```python
from build123d import *

# Parameters (mm, degrees)
F1_DEPTH = 1.7
F2_DEPTH = 7
F3_DEPTH = 22


with BuildPart() as f1:
    # F0 (on Top) → F1 (new body)
    with BuildSketch(Plane.XY):
        with BuildLine():
            Line((-22, -24), (-16, -24))
            Line((-16, -24), (-16, -14))
            ThreePointArc((-16, -14), (-11.313708, -2.686292), (0, 2))
            Line((0, 2), (128, 2))
            ThreePointArc((128, 2), (139.313708, -2.686292), (144, -14))
            Line((144, -14), (144, -24))
            Line((144, -24), (150, -24))
            Line((150, -24), (150, -14))
            ThreePointArc((150, -14), (143.556349, 1.556349), (128, 8))
            Line((128, 8), (0, 8))
            ThreePointArc((0, 8), (-15.556349, 1.556349), (-22, -14))
            Line((-22, -14), (-22, -24))
        make_face()
    extrude(amount=F1_DEPTH)

    # F0 (on Top) → F2 (join)
    with BuildSketch(Plane.XY):
        with BuildLine():
            ThreePointArc((-14, -14), (-9.899495, -4.100505), (0, 0))
            Line((0, 0), (128, 0))
            ThreePointArc((128, 0), (137.899495, -4.100505), (142, -14))
            Line((142, -14), (142, -24))
            Line((142, -24), (144, -24))
            Line((144, -24), (144, -14))
            ThreePointArc((144, -14), (139.313708, -2.686292), (128, 2))
            Line((128, 2), (0, 2))
            ThreePointArc((0, 2), (-11.313708, -2.686292), (-16, -14))
            Line((-16, -14), (-16, -24))
            Line((-16, -24), (-14, -24))
            Line((-14, -24), (-14, -14))
        make_face()
    extrude(amount=F2_DEPTH)

    # F0 (on Top) → F3 (join)
    with BuildSketch(Plane.XY):
        with BuildLine():
            Line((-24, -24), (-22, -24))
            Line((-22, -24), (-22, -14))
            ThreePointArc((-22, -14), (-15.556349, 1.556349), (0, 8))
            Line((0, 8), (128, 8))
            ThreePointArc((128, 8), (143.556349, 1.556349), (150, -14))
            Line((150, -14), (150, -24))
            Line((150, -24), (152, -24))
            Line((152, -24), (152, -14))
            ThreePointArc((152, -14), (144.970563, 2.970563), (128, 10))
            Line((128, 10), (0, 10))
            ThreePointArc((0, 10), (-16.970563, 2.970563), (-24, -14))
            Line((-24, -14), (-24, -24))
        make_face()
    extrude(amount=F3_DEPTH)


solid = f1.part
```
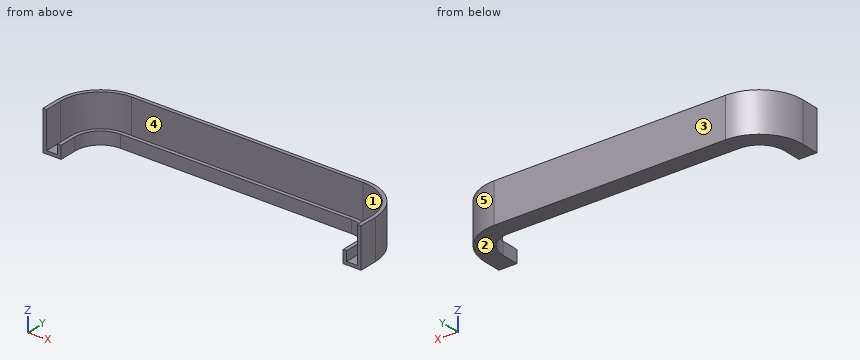
Geometry: final body of the model. Coordinates: model frame, mm. Face numbers are marked on the shaded views. A direction names the side the tool comes from. Coordinates: 2 decimals unless noted, no trailing zeros. Order: outer loops, then holes, each group sorted by start corner. A loop starts at its lowest first (then second) coordinate and runs counter-clockwise, first axis right, second up. Notation, with made-up numbers: M 88.5,-10 L 99.5,-10 A29 cw 99.5,18 Z; hole C 70,78 d6. An arc over 180 degrees is marked long. Answer in a Markdown table with one row per item. Add a question column.
Q1. Mould query, pull axis Y, two halves, no side actions, for the marked faces 1, 2 and 3. Classes: released by +Y, released by -Y, zero draft, split by the parting line, or undercut.
Q2. Section query D-D on y = -6. Return the cut outline in (x, z), and give its area (3 significant figures).
Q3. Reachability of the marked faces 4 and 5 from +Z, -Z, +X, -X, +Y, -Y: full face, straight path, thin tool, end or side. Return the list, or none.
Q4. Line query: L1, parallel to X at y = -14, z = 5; L2, parallel to X at y = -11, z = 6.5; L3, parallel to X at y = -21.5, z = 1. Output: solid intervals per line, ascending.
Q5. Section query A-A on y = -15.5. Return the cut outline in (x, z), and give its area (3 significant figures).
Q6. Section query C-C on x = 15. Return the cut outline in (y, z), and give its area (3 significant figures).
Q7. Section query B-B on z = 16.5. Return the cut outline in (x, y), and give its area (3 significant figures).
Q8. Contact query for flat-ended pins moving along their axis: P1, Ø1.5, axis at y = 3.5, z = 11.5, coming from the +X side; P2, Ø2, axis at y = 1, z = 19, coming from the +X side; P3, Ø6, axis at x = 72.5, z = 7, coming from the -Y side. Output: stop coordinate, or through.
Completed:
| question | item | result |
|---|---|---|
| 1 | face 1 | undercut |
| 1 | face 2 | zero draft |
| 1 | face 3 | released by +Y |
| 2 | outline | M -22.63,0 L -11.49,0 L -11.49,7 L -13.86,7 L -13.86,1.7 L -20.49,1.7 L -20.49,22 L -22.63,22 Z; M 139.49,0 L 150.63,0 L 150.63,22 L 148.49,22 L 148.49,1.7 L 141.86,1.7 L 141.86,7 L 139.49,7 Z |
| 2 | area | 150 mm2 |
| 3 | face 4 | +Z |
| 3 | face 5 | +Z, -Z, +X, +Y |
| 4 | L1 | x = -24 to -22, -16 to -14, 142 to 144, 150 to 152 |
| 4 | L2 | x = -23.81 to -21.79, -15.72 to -13.67, 141.67 to 143.72, 149.79 to 151.81 |
| 4 | L3 | x = -24 to -14, 142 to 152 |
| 5 | outline | M -24,0 L -14,0 L -14,7 L -16,7 L -16,1.7 L -22,1.7 L -22,22 L -24,22 Z; M 142,0 L 152,0 L 152,22 L 150,22 L 150,1.7 L 144,1.7 L 144,7 L 142,7 Z |
| 5 | area | 136 mm2 |
| 6 | outline | M 0,0 L 10,0 L 10,22 L 8,22 L 8,1.7 L 2,1.7 L 2,7 L 0,7 Z |
| 6 | area | 68.2 mm2 |
| 7 | outline | M -24,-24 L -22,-24 L -22,-14 A22 cw 0,8 L 128,8 A22 cw 150,-14 L 150,-24 L 152,-24 L 152,-14 A24 ccw 128,10 L 0,10 A24 ccw -24,-14 Z |
| 7 | area | 441 mm2 |
| 8 | P1 | stops at x = 145.19 |
| 8 | P2 | stops at x = 147.49 |
| 8 | P3 | stops at y = 0 |
